Part print with two shaded views. Sizes in mm from the minimum x, y, z corner. A direction names the side the tool comes from. Give positions to 0.01 mm unless a question says otherwise; leave off trailing zeros. Order: outer loops, then holes, each group sorted by start corner. A loop starts at its lowest first (then second) coordinate and runs counter-clockwise, first axis right, second up.
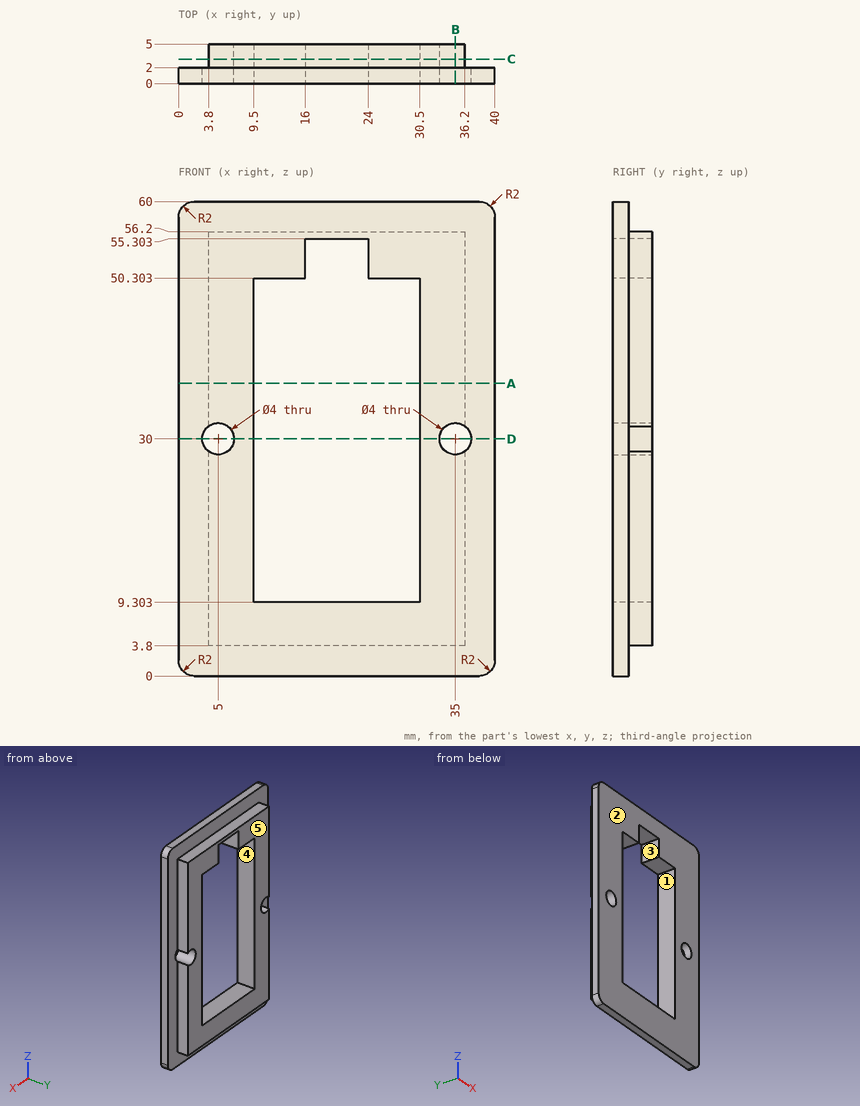
Item 1: Drop flat-ended pins along their axis: pin 1 Ø2.5 at (y, z) = (4, 19.5) entering from +X; pin 2 Ø1 at (y, z) = (3.5, 35) entering from -X; pin 3 Ø0.9 at (x, y) = (27, 3) entering from -Z; pin 4 Ø3 at (x, z) = (35, 30) entering from +Y. Give the stop position or say it passes through.
Item 2: Tool access for the marked faces 1 and 2: list every direction of +Z, -Z, +X, -X, +Y, -Y with a clear straight run to the whole face (end or side of a thin tool).
Item 3: Slice it at C-C (y = 3.1). Give the cut face in (x, z), and give its area (3 significant figures).
Item 4: Two-plate mould, pull along X, no slides. Class the marked faces 3, 4 and 5: released by +X, released by -X, zero draft, split by the parting line, or undercut.
Item 5: Slice it at A-A (z = 37). Give the cut face in (x, y), and give its area (3 significant figures).
Item 6: Slice it at D-D (z = 30). Give the cut face in (x, y), and give its area (3 significant figures).
Item 7: Wall check: L1, parallel to Z at x = 5, y = 2.65; L2, parallel to Z at x = 35, y = 1.5; L3, parallel to X at y = 1.7, z = 16.5. Give the ranges that are in metal, low to high.
Item 8: Slice it at B-B (x = 35). Give the cut face in (y, z).
A:
1. pin 1: stops at x = 36.2
1. pin 2: stops at x = 3.8
1. pin 3: stops at z = 3.8
1. pin 4: passes through
2. face 1: +Y, -Y
2. face 2: +Z, -Z, +X, -X, -Y
3. outline: (3.8, 3.8) - (36.2, 3.8) - (36.2, 28.4) arc R2 cw (long way) to (36.2, 31.6) - (36.2, 56.2) - (3.8, 56.2) - (3.8, 31.6) arc R2 cw (long way) to (3.8, 28.4) - close; hole (9.5, 9.3) - (30.5, 9.3) - (30.5, 50.3) - (24, 50.3) - (24, 55.3) - (16, 55.3) - (16, 50.3) - (9.5, 50.3) - close
3. area: 775 mm2
4. face 3: undercut
4. face 4: undercut
4. face 5: zero draft
5. outline: (0, 0) - (9.5, 0) - (9.5, 5) - (3.8, 5) - (3.8, 2) - (0, 2) - close; (30.5, 0) - (40, 0) - (40, 2) - (36.2, 2) - (36.2, 5) - (30.5, 5) - close
5. area: 72.2 mm2
6. outline: (0, 0) - (3, 0) - (3, 2) - (0, 2) - close; (7, 0) - (9.5, 0) - (9.5, 5) - (7, 5) - close; (30.5, 0) - (33, 0) - (33, 5) - (30.5, 5) - close; (37, 0) - (40, 0) - (40, 2) - (37, 2) - close
6. area: 37.0 mm2
7. L1: z = 3.8 to 28, 32 to 56.2
7. L2: z = 0 to 28, 32 to 60
7. L3: x = 0 to 9.5, 30.5 to 40
8. outline: (0, 0) - (2, 0) - (2, 3.8) - (5, 3.8) - (5, 28) - (0, 28) - close; (0, 32) - (5, 32) - (5, 56.2) - (2, 56.2) - (2, 60) - (0, 60) - close
